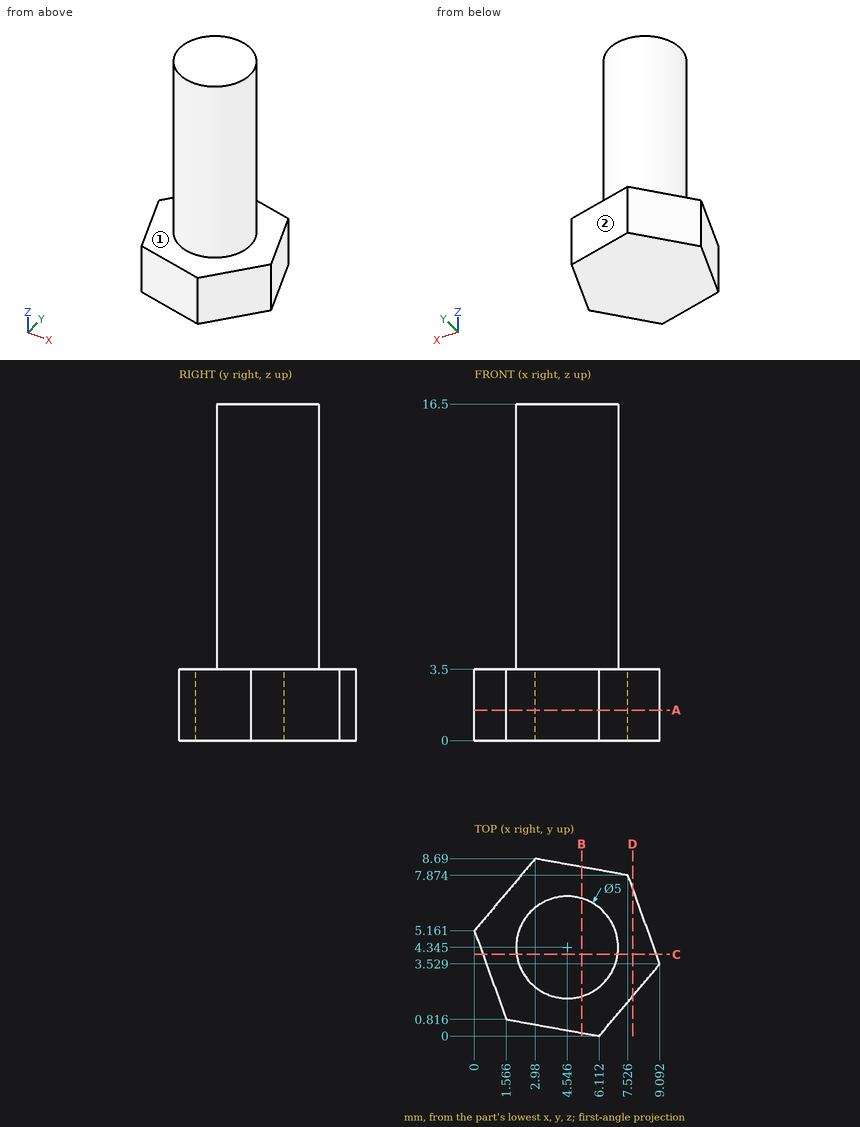
Geometry check sheet. Reference: drawing and pictorial views, mm from the part's lowest x, y, z. A direction names the side the tool comes from. Coordinates: 2 decimals unless noted, no trailing zeros. Loops run counter-clockwise (first coordinate to the right, second up) from the corner with the lowest first, then second, coordinate; pieces in that order, holes last.
1) Access from +Z, -Z, +X, -X, +Y, -Y to the whole of each face (thin tool, end or side, straight path). Record for the marked faces 1 and 2.
2) Sectioned sample at C-C (y = 4). Record the boundary of the cut face in (x, z).
3) Sectioned sample at D-D (x = 7.75). Record the boundary of the cut face in (y, z).
4) Gauge pin test, flat ends, axial feed: pin 1 (4 mm diameter, centred on x = 6, z = 12.5, fed in from +Y) (1 decimal); pin 2 (2 mm diameter, centred on y = 6, z = 10, fed in from +X); pin 3 (1.5 mm diameter, centred on x = 6.5, z = 13.5, fed in from -Y) (1 decimal). Record the tip position at first contact, or that the pin passes through.
5) Sectioned sample at A-A (z = 1.5). Record the boundary of the cut face in (x, y) (1 decimal).
6) Sectioned sample at B-B (x = 5.25). Record the boundary of the cut face in (y, z) (1 decimal).
7) Material ranges on probe 1 along Z at (x, y) = (7, 1.75); probe 2 along X at (y, z) = (4.25, 8.5) (1 decimal); probe 3 along X at (y, z) = (5.25, 10) (1 decimal), recorded low to high.
Check sheet entries:
1. face 1: +Z
1. face 2: +Z, -Z, +X, +Y
2. outline: (0.42, 0) - (8.92, 0) - (8.92, 3.5) - (7.02, 3.5) - (7.02, 16.5) - (2.07, 16.5) - (2.07, 3.5) - (0.42, 3.5) - close
3. outline: (1.94, 0) - (7.25, 0) - (7.25, 3.5) - (1.94, 3.5) - close
4. pin 1: stops at y = 6.8
4. pin 2: stops at x = 6.96
4. pin 3: stops at y = 2.2
5. outline: (0, 5.2) - (1.6, 0.8) - (6.1, 0) - (9.1, 3.5) - (7.5, 7.9) - (3, 8.7) - close
6. outline: (0.2, 0) - (8.3, 0) - (8.3, 3.5) - (6.7, 3.5) - (6.7, 16.5) - (1.9, 16.5) - (1.9, 3.5) - (0.2, 3.5) - close
7. probe 1: z = 0 to 3.5
7. probe 2: x = 2 to 7
7. probe 3: x = 2.2 to 6.9
